Geometry check sheet. Reference: the model listing, model coordinates, mm. A direction names the side the tool comes from. Round coordinates to 2 decimals unless told otherwise and drop trailing zeros. Order: outer loops, then holes, each group sorted by start corner. A loop starts at its lowest first (then second) coordinate and runs counter-clockwise, first axis right, second up. Notation, with made-up numbers: (-37.5, -3) - (19.5, -3) arc R23 ccw to (19.5, 19) - close; hole circle Ø11 at (79, 8.5). An arc over 180 degrees is marked (long way). One line per question, with ' | ' between items. Start each with the question number.
Q1. Sectioned sample at C-C, the plane x = -45. Enter the section's corners in (y, z), then the cut area to 3 significant figures.
Q2. Mould release check, pull along X, two halves, no side actions. Record for faces 1 (the face through (-9.732, 29, 62)), 2 (the face through (-44, 30, -4)), 3 (the face through (-46, 28, 57)): +X half, -X half, draft (parallel to the pull), parting line (faces both ways), or undercut.
Q3. Sectioned sample at D-D, the plane y = 30. Enter the section's corners in (x, z).
Q4. Gauge pin test, flat ends, axial feed: P1, Ø6, axis at x = 8.5, y = 5.5, coming from the +Z side; P2, Ø3, axis at y = 25, z = -2.5, coming from the +X side; P3, Ø5, axis at x = -0.5, z = 40, coming from the -Y side; P4, Ø20.5, axis at x = -41, z = 46, coming from the -Y side. Record the tip position at first contact, or that the pin passes through.
Q5. Sectioned sample at A-A, the plane y = 6.5. Enter the section's corners in (x, z), then the cut area to 3 significant figures.
Q6. Sectioned sample at B-B, the plane z = 6.5. Enter the section's corners in (x, y), then the cut area to 3 significant figures.
Q7. Material ranges on line 1 along Z through (x, y) = (-15, 28); line 2 along Z through (x, y) = (-48, 25); line 3 along X through (y, z) = (27, 18), recorded low to high.
Q8. Tool access check on faces 4 (the face through (-15, 26, 8)), 5 (the face through (-9.732, 29, -2)), 6 (the face through (-7, 38.402, 30)), 7 (the face through (12.268, 1, 30)). Record the directions out of +Z, -Z, +X, -X, +Y, -Y that give a thin tool (end or side, any length) a straight path to the whole face; none if there is none.
```python
from build123d import *

# Parameters (mm, degrees)
EXTRUDE_1_DEPTH     = 60
SKETCH_2_W          = 7
SKETCH_2_H          = 20
EXTRUDE_2_DEPTH     = 54
SKETCH_3_W          = 4
SKETCH_3_H          = 20
EXTRUDE_3_DEPTH     = 10
SKETCH_4_W          = 68
SKETCH_4_H          = 41.598220465
EXTRUDE_4_DEPTH     = 6
SKETCH_5_W          = 44
SKETCH_5_H          = 25.180333828
CUT_EXTRUDE_1_DEPTH = 10


with BuildPart() as part:
    # 草图1 → 凸台-拉伸1 (new body)
    with BuildSketch(Plane.XY):
        Polygon((-19.732146976, -1.598220465), (-11.732146976, -1.598220465), (-11.732146976, 3.401779535), (-15.732146976, 3.401779535), (-15.732146976, 8.401779535), (16.267853024, 8.401779535), (16.267853024, 3.401779535), (12.267853024, 3.401779535), (12.267853024, -1.598220465), (20.267853024, -1.598220465), (20.267853024, 38.401779535), (-19.732146976, 38.401779535), align=None)
    extrude(amount=EXTRUDE_1_DEPTH)

    # 草图2 → 凸台-拉伸2 (add)
    with BuildSketch(Plane.ZY.offset(19.732146976)):
        with Locations((-0.5, 28.401779535)):
            Rectangle(SKETCH_2_W, SKETCH_2_H)
        with Locations((60.5, 28.401779535)):
            Rectangle(SKETCH_2_W, SKETCH_2_H)
    extrude(amount=EXTRUDE_2_DEPTH)

    # 草图3 → 凸台-拉伸3 (add)
    with BuildSketch(Plane(origin=(-19.732146976, 0, 0), x_dir=(0, 0, -1), z_dir=(1, 0, 0))):
        with Locations((-62, 28.401779535)):
            Rectangle(SKETCH_3_W, SKETCH_3_H)
        with Locations((2, 28.401779535)):
            Rectangle(SKETCH_3_W, SKETCH_3_H)
    extrude(amount=EXTRUDE_3_DEPTH)

    # 草图4 → 凸台-拉伸4 (add)
    with BuildSketch(Plane.ZY.offset(73.732146976)):
        with Locations((30, 39.200889768)):
            Rectangle(SKETCH_4_W, SKETCH_4_H)
    extrude(amount=EXTRUDE_4_DEPTH)

    # 草图5 → 切除-拉伸1 (cut)
    with BuildSketch(Plane.ZY.offset(19.732146976)):
        with Locations((30, 25.991946449)):
            Rectangle(SKETCH_5_W, SKETCH_5_H)
    extrude(amount=-CUT_EXTRUDE_1_DEPTH, mode=Mode.SUBTRACT)


solid = part.part
```
Determined:
1) outline: (18.4, -4) - (38.4, -4) - (38.4, 3) - (18.4, 3) - close; (18.4, 57) - (38.4, 57) - (38.4, 64) - (18.4, 64) - close | area: 280 mm2
2) face 1: +X half | face 2: draft | face 3: undercut
3) outline: (-79.73, -4) - (-9.73, -4) - (-9.73, 0) - (20.27, 0) - (20.27, 60) - (-9.73, 60) - (-9.73, 64) - (-79.73, 64) - close; hole (-73.73, 3) - (-19.73, 3) - (-19.73, 8) - (-9.73, 8) - (-9.73, 52) - (-19.73, 52) - (-19.73, 57) - (-73.73, 57) - close
4) P1: stops at z = 60 | P2: stops at x = -9.73 | P3: stops at y = 8.4 | P4: passes through
5) outline: (-19.73, 0) - (-15.73, 0) - (-15.73, 60) - (-19.73, 60) - close; (16.27, 0) - (20.27, 0) - (20.27, 60) - (16.27, 60) - close | area: 480 mm2
6) outline: (-79.73, 18.4) - (-73.73, 18.4) - (-73.73, 60) - (-79.73, 60) - close; (-19.73, -1.6) - (-11.73, -1.6) - (-11.73, 3.4) - (-15.73, 3.4) - (-15.73, 8.4) - (16.27, 8.4) - (16.27, 3.4) - (12.27, 3.4) - (12.27, -1.6) - (20.27, -1.6) - (20.27, 38.4) - (-19.73, 38.4) - close | area: 1,570 mm2
7) line 1: z = -4 to 8, 52 to 64 | line 2: z = -4 to 3, 57 to 64 | line 3: x = -79.73 to -73.73, -9.73 to 20.27
8) face 4: +Y | face 5: -Z, +X, +Y, -Y | face 6: +Z, -Z, +X, +Y | face 7: +Z, -Z, -Y
